from build123d import *

# Parameters (mm, degrees)
SKETCH005_W     = 25.4
SKETCH005_H     = 25.4
PAD002_DEPTH    = 609.6
SKETCH006_R     = 4
POCKET003_DEPTH = 25.401
POCKET004_DEPTH = 25.401
POCKET007_DEPTH = 25.401
SKETCH012_R     = 8.255
POCKET008_DEPTH = 5.08
SKETCH013_R     = 1.5875
POCKET009_DEPTH = 25.401


with BuildPart() as part:
    # Sketch005 → Pad002 (new body)
    with BuildSketch(Plane.XY):
        Rectangle(SKETCH005_W, SKETCH005_H)
        with BuildLine():
            ThreePointArc((-9.525, -6.35), (-8.595064, -8.595064), (-6.35, -9.525))
            Line((6.35, -9.525), (-6.35, -9.525))
            ThreePointArc((6.35, -9.525), (8.595064, -8.595064), (9.525, -6.35))
            Line((9.525, 6.35), (9.525, -6.35))
            ThreePointArc((9.525, 6.35), (8.595064, 8.595064), (6.35, 9.525))
            Line((-6.35, 9.525), (6.35, 9.525))
            ThreePointArc((-6.35, 9.525), (-8.595064, 8.595064), (-9.525, 6.35))
            Line((-9.525, -6.35), (-9.525, 6.35))
        make_face(mode=Mode.SUBTRACT)
    extrude(amount=PAD002_DEPTH)

    # Sketch006 (on Face3 of Pad002) → Pocket003 (cut, through all)
    with BuildSketch(Plane.YZ.offset(12.7)):
        with Locations((0, 584.2)):
            Circle(SKETCH006_R)
        with Locations((0, 533.4)):
            Circle(SKETCH006_R)
    extrude(amount=-POCKET003_DEPTH, mode=Mode.SUBTRACT)

    # Sketch007 (on Face2 of Pocket003) → Pocket004 (cut, through all)
    with BuildSketch(Plane.XZ.offset(12.7)):
        Polygon((12.7, 25.4), (-12.7, 0), (12.7, 0), align=None)
    extrude(amount=-POCKET004_DEPTH, mode=Mode.SUBTRACT)

    # Sketch011 (on Face1 of Pocket004) → Pocket007 (cut, through all)
    with BuildSketch(Plane(origin=(-12.7, 0, 0), x_dir=(0, -1, 0), z_dir=(-1, 0, 0))):
        with BuildLine():
            ThreePointArc((-7.62, 544.5125), (-6.225096, 541.144904), (-2.8575, 539.75))
            Line((2.8575, 539.75), (-2.8575, 539.75))
            ThreePointArc((2.8575, 539.75), (6.225096, 541.144904), (7.62, 544.5125))
            Line((7.62, 573.0875), (7.62, 544.5125))
            ThreePointArc((7.62, 573.0875), (6.225096, 576.455096), (2.8575, 577.85))
            Line((-2.8575, 577.85), (2.8575, 577.85))
            ThreePointArc((-2.8575, 577.85), (-6.225096, 576.455096), (-7.62, 573.0875))
            Line((-7.62, 544.5125), (-7.62, 573.0875))
        make_face()
    extrude(amount=-POCKET007_DEPTH, mode=Mode.SUBTRACT)

    # Sketch012 (on Face2 of Pocket007) → Pocket008 (cut)
    with BuildSketch(Plane.XZ.offset(12.7)):
        with Locations((0, 558.8)):
            Circle(SKETCH012_R)
    extrude(amount=-POCKET008_DEPTH, mode=Mode.SUBTRACT)

    # Sketch013 (on Face2 of Pocket008) → Pocket009 (cut, through all)
    with BuildSketch(Plane.XZ.offset(12.7)):
        with Locations((0, 558.8)):
            Circle(SKETCH013_R)
    extrude(amount=-POCKET009_DEPTH, mode=Mode.SUBTRACT)


solid = part.part
Part model, mm, in its own coordinate system. A direction names the side the tool comes from. Give positions to 0.01 mm unless a question says otherwise; leave off trailing zeros. Loops run counter-clockwise (first coordinate to the right, second up) from the corner with the lowest first, then second, coordinate; pieces in that order, holes last.
(1) Pull direction Y, two halves, no side cores. Call faces 1 (the flat face through (-9.525, 0, 268)), 2 (the flat face through (0, -9.525, 587)), 3 (the flat face through (0, -12.7, 301)), 4 (the flat face through (0, 12.7, 301)): pulls with the +Y half, pulls with the -Y half, needs draft (parallel to the pull), parting line crosses it, or undercut.
Return value:
face 1: undercut
face 2: undercut
face 3: pulls with the -Y half
face 4: pulls with the +Y half
(2) Drill centre lines: line 1 along X through (y, z) = (0.75, 368) (3 decimals); line 2 along Y through (x, z) = (7.5, 249). Where is each one in solid material? Low to high.
Return value:
line 1: x = -12.7 to -9.525, 9.525 to 12.7
line 2: y = -12.7 to -9.31, 9.31 to 12.7
(3) Band-saw the part on A-A (z = 73). Write the cut outline in (x, y) (3 decimals).
Return value:
outline: (-12.7, -12.7) - (12.7, -12.7) - (12.7, 12.7) - (-12.7, 12.7) - close; hole (-9.525, -6.35) arc R3.175 ccw to (-6.35, -9.525) - (6.35, -9.525) arc R3.175 ccw to (9.525, -6.35) - (9.525, 6.35) arc R3.175 ccw to (6.35, 9.525) - (-6.35, 9.525) arc R3.175 ccw to (-9.525, 6.35) - close
(4) 3-axis set-ups, long thin cutter, end or side, ignore diameter. For faces 5 (the flat face through (9.525, 0, 593)), 6 (the flat face through (-12.7, 0, 301)), 7 (the cylindrical face through (-8.247, -10.822, 559.163)): which of +Z, -Z, +X, -X, +Y, -Y reach the whole face in a straight line?
Return value:
face 5: +Z, -Z
face 6: +Z, -Z, -X, +Y, -Y
face 7: -Y
(5) Pin check, flat tips, straight feed: pin 1 (1.6 mm diameter, centred on x = -11.5, y = -0.5, fed in from -Z); pin 2 (12 mm diameter, centred on x = -4, y = -1.5, fed in from -Z); pin 3 (5 mm diameter, centred on x = -9.5, y = 4.5, fed in from -Z). Stop position of each tip, or through.
Return value:
pin 1: stops at z = 0.4
pin 2: stops at z = 2.7
pin 3: stops at z = 0.7
